from build123d import *

# Parameters (mm, degrees)
BOSS_EXTRUDE1_DEPTH = 7.5
FILLET1_R           = 3.75
FILLET2_R           = 3.75


# Some blends are built 0.0001 mm under size
with BuildPart() as part:
    # Sketch2 → Boss-Extrude1 (new body)
    with BuildSketch(Plane(origin=(0, 0, 0), x_dir=(1, 0, 0), z_dir=(0, 1, 0))):
        Polygon((-54.865, 27.5), (-54.865, -27.5), (-47.365, -27.5), (-47.365, -5), (47.365, -5), (47.365, -27.5), (54.865, -27.5), (54.865, 27.5), (47.365, 27.5), (47.365, 5), (-47.365, 5), (-47.365, 27.5), align=None)
    extrude(amount=BOSS_EXTRUDE1_DEPTH)

    # Fillet1
    fillet1_edges = [part.edges().sort_by_distance(p)[0] for p in [
        (0, 7.5, 5),
        (-54.865, 0, 0),
        (-47.365, 0, -16.25),
        (0, 0, -5),
        (47.365, 0, -16.25),
        (47.365, 7.5, 16.25),
        (54.865, 0, 0),
        (47.365, 0, 16.25),
        (0, 0, 5),
        (-47.365, 0, 16.25),
        (54.865, 7.5, 0),
        (-54.865, 3.75, 27.5),
        (-54.865, 3.75, -27.5),
        (-47.365, 3.75, -27.5),
        (-47.365, 3.75, -5),
        (47.365, 3.75, -5),
        (47.365, 3.75, -27.5),
        (54.865, 3.75, -27.5),
        (54.865, 3.75, 27.5),
        (47.365, 3.75, 27.5),
        (47.365, 3.75, 5),
        (-47.365, 3.75, 5),
        (-47.365, 3.75, 27.5),
        (47.365, 7.5, -16.25),
        (0, 7.5, -5),
        (-47.365, 7.5, -16.25),
        (-54.865, 7.5, 0),
        (-47.365, 7.5, 16.25),
    ]]
    fillet(fillet1_edges, radius=FILLET1_R - 0.0001)  # a hair under: the kernel refuses the full size

    # Fillet2
    # the kernel refuses this fillet: 3.75 mm, written as the material it takes off along each edge
    with BuildSketch(Plane(origin=(-47.365, 3.75, -23.75), x_dir=(0, 0, -1), z_dir=(0, -1, 0))) as fillet2_piece_1:
        with BuildLine():
            CenterArc((0.0001, -3.7499), 3.7499, 0, 90)
            Line((3.75, -3.7499), (3.75, 0))
            Line((3.75, 0), (0.0001, 0))
        make_face()
    revolve(axis=Axis((-47.365, 3.75, -23.75), (1, 0, 0)), revolution_arc=90, mode=Mode.SUBTRACT)
    with BuildSketch(Plane(origin=(-47.365, 3.75, -23.75), x_dir=(0, -1, 0), z_dir=(0, 0, 1))) as fillet2_piece_2:
        with BuildLine():
            CenterArc((0.0001, -3.7499), 3.7499, 0, 90)
            Line((3.75, -3.7499), (3.75, 0))
            Line((3.75, 0), (0.0001, 0))
        make_face()
    revolve(axis=Axis((-47.365, 3.75, -23.75), (1, 0, 0)), revolution_arc=90, mode=Mode.SUBTRACT)
    with BuildSketch(Plane(origin=(-54.865, 3.75, 23.75), x_dir=(0, 0, 1), z_dir=(0, -1, 0))) as fillet2_piece_3:
        with BuildLine():
            CenterArc((0.0001, -3.7499), 3.7499, 0, 90)
            Line((3.75, -3.7499), (3.75, 0))
            Line((3.75, 0), (0.0001, 0))
        make_face()
    revolve(axis=Axis((-54.865, 3.75, 23.75), (-1, 0, 0)), revolution_arc=90, mode=Mode.SUBTRACT)
    with BuildSketch(Plane(origin=(-54.865, 3.75, 23.75), x_dir=(0, -1, 0), z_dir=(0, 0, -1))) as fillet2_piece_4:
        with BuildLine():
            CenterArc((0.0001, -3.7499), 3.7499, 0, 90)
            Line((3.75, -3.7499), (3.75, 0))
            Line((3.75, 0), (0.0001, 0))
        make_face()
    revolve(axis=Axis((-54.865, 3.75, 23.75), (-1, 0, 0)), revolution_arc=90, mode=Mode.SUBTRACT)
    with BuildSketch(Plane(origin=(47.365, 3.75, 23.75), x_dir=(0, -1, 0), z_dir=(0, 0, -1))) as fillet2_piece_5:
        with BuildLine():
            CenterArc((0.0001, -3.7499), 3.7499, 0, 90)
            Line((3.75, -3.7499), (3.75, 0))
            Line((3.75, 0), (0.0001, 0))
        make_face()
    revolve(axis=Axis((47.365, 3.75, 23.75), (-1, 0, 0)), revolution_arc=90, mode=Mode.SUBTRACT)
    with BuildSketch(Plane(origin=(47.365, 3.75, 23.75), x_dir=(0, 0, 1), z_dir=(0, -1, 0))) as fillet2_piece_6:
        with BuildLine():
            CenterArc((0.0001, -3.7499), 3.7499, 0, 90)
            Line((3.75, -3.7499), (3.75, 0))
            Line((3.75, 0), (0.0001, 0))
        make_face()
    revolve(axis=Axis((47.365, 3.75, 23.75), (-1, 0, 0)), revolution_arc=90, mode=Mode.SUBTRACT)
    with BuildSketch(Plane(origin=(54.865, 3.75, -23.75), x_dir=(0, -1, 0), z_dir=(0, 0, 1))) as fillet2_piece_7:
        with BuildLine():
            CenterArc((0.0001, -3.7499), 3.7499, 0, 90)
            Line((3.75, -3.7499), (3.75, 0))
            Line((3.75, 0), (0.0001, 0))
        make_face()
    revolve(axis=Axis((54.865, 3.75, -23.75), (1, 0, 0)), revolution_arc=90, mode=Mode.SUBTRACT)
    with BuildSketch(Plane(origin=(54.865, 3.75, -23.75), x_dir=(0, 0, -1), z_dir=(0, -1, 0))) as fillet2_piece_8:
        with BuildLine():
            CenterArc((0.0001, -3.7499), 3.7499, 0, 90)
            Line((3.75, -3.7499), (3.75, 0))
            Line((3.75, 0), (0.0001, 0))
        make_face()
    revolve(axis=Axis((54.865, 3.75, -23.75), (1, 0, 0)), revolution_arc=90, mode=Mode.SUBTRACT)
    with BuildSketch(Plane(origin=(-54.865, 3.75, -23.75), x_dir=(0, 1, 0), z_dir=(0, 0, 1))) as fillet2_piece_9:
        with BuildLine():
            CenterArc((0.0001, -3.7499), 3.7499, 0, 90)
            Line((3.75, -3.7499), (3.75, 0))
            Line((3.75, 0), (0.0001, 0))
        make_face()
    revolve(axis=Axis((-54.865, 3.75, -23.75), (-1, 0, 0)), revolution_arc=90, mode=Mode.SUBTRACT)
    with BuildSketch(Plane(origin=(-54.865, 3.75, -23.75), x_dir=(0, 0, -1), z_dir=(0, 1, 0))) as fillet2_piece_10:
        with BuildLine():
            CenterArc((0.0001, -3.7499), 3.7499, 0, 90)
            Line((3.75, -3.7499), (3.75, 0))
            Line((3.75, 0), (0.0001, 0))
        make_face()
    revolve(axis=Axis((-54.865, 3.75, -23.75), (-1, 0, 0)), revolution_arc=90, mode=Mode.SUBTRACT)
    with BuildSketch(Plane(origin=(-47.365, 3.75, 23.75), x_dir=(0, 1, 0), z_dir=(0, 0, -1))) as fillet2_piece_11:
        with BuildLine():
            CenterArc((0.0001, -3.7499), 3.7499, 0, 90)
            Line((3.75, -3.7499), (3.75, 0))
            Line((3.75, 0), (0.0001, 0))
        make_face()
    revolve(axis=Axis((-47.365, 3.75, 23.75), (1, 0, 0)), revolution_arc=90, mode=Mode.SUBTRACT)
    with BuildSketch(Plane(origin=(-47.365, 3.75, 23.75), x_dir=(0, 0, 1), z_dir=(0, 1, 0))) as fillet2_piece_12:
        with BuildLine():
            CenterArc((0.0001, -3.7499), 3.7499, 0, 90)
            Line((3.75, -3.7499), (3.75, 0))
            Line((3.75, 0), (0.0001, 0))
        make_face()
    revolve(axis=Axis((-47.365, 3.75, 23.75), (1, 0, 0)), revolution_arc=90, mode=Mode.SUBTRACT)
    with BuildSketch(Plane(origin=(54.865, 3.75, 23.75), x_dir=(0, 0, 1), z_dir=(0, 1, 0))) as fillet2_piece_13:
        with BuildLine():
            CenterArc((0.0001, -3.7499), 3.7499, 0, 90)
            Line((3.75, -3.7499), (3.75, 0))
            Line((3.75, 0), (0.0001, 0))
        make_face()
    revolve(axis=Axis((54.865, 3.75, 23.75), (1, 0, 0)), revolution_arc=90, mode=Mode.SUBTRACT)
    with BuildSketch(Plane(origin=(54.865, 3.75, 23.75), x_dir=(0, 1, 0), z_dir=(0, 0, -1))) as fillet2_piece_14:
        with BuildLine():
            CenterArc((0.0001, -3.7499), 3.7499, 0, 90)
            Line((3.75, -3.7499), (3.75, 0))
            Line((3.75, 0), (0.0001, 0))
        make_face()
    revolve(axis=Axis((54.865, 3.75, 23.75), (1, 0, 0)), revolution_arc=90, mode=Mode.SUBTRACT)
    with BuildSketch(Plane(origin=(47.365, 3.75, -23.75), x_dir=(0, 0, -1), z_dir=(0, 1, 0))) as fillet2_piece_15:
        with BuildLine():
            CenterArc((0.0001, -3.7499), 3.7499, 0, 90)
            Line((3.75, -3.7499), (3.75, 0))
            Line((3.75, 0), (0.0001, 0))
        make_face()
    revolve(axis=Axis((47.365, 3.75, -23.75), (-1, 0, 0)), revolution_arc=90, mode=Mode.SUBTRACT)
    with BuildSketch(Plane(origin=(47.365, 3.75, -23.75), x_dir=(0, 1, 0), z_dir=(0, 0, 1))) as fillet2_piece_16:
        with BuildLine():
            CenterArc((0.0001, -3.7499), 3.7499, 0, 90)
            Line((3.75, -3.7499), (3.75, 0))
            Line((3.75, 0), (0.0001, 0))
        make_face()
    revolve(axis=Axis((47.365, 3.75, -23.75), (-1, 0, 0)), revolution_arc=90, mode=Mode.SUBTRACT)
    with BuildSketch(Plane(origin=(54.865, 7.5, -27.5), x_dir=(0, 0, 1), z_dir=(-1, 0, 0)), Plane(origin=(47.365, 7.5, 27.5), x_dir=(0, 0, -1), z_dir=(1, 0, 0))) as fillet2_piece_17:
        with BuildLine():
            CenterArc((FILLET2_R, -FILLET2_R), FILLET2_R, 90, 90)
            Line((0, -FILLET2_R), (0, 0))
            Line((0, 0), (FILLET2_R, 0))
        make_face()
    extrude(amount=7.5, mode=Mode.SUBTRACT)
    with BuildSketch(Plane(origin=(54.865, 0, -27.5), x_dir=(0, 0, 1), z_dir=(-1, 0, 0)), Plane(origin=(47.365, 0, 27.5), x_dir=(0, 0, -1), z_dir=(1, 0, 0)), Plane(origin=(-54.865, 0, 27.5), x_dir=(0, 0, -1), z_dir=(1, 0, 0)), Plane(origin=(-54.865, 7.5, 27.5), x_dir=(0, -1, 0), z_dir=(1, 0, 0)), Plane(origin=(-47.365, 0, -27.5), x_dir=(0, 0, 1), z_dir=(-1, 0, 0)), Plane(origin=(-47.365, 7.5, -27.5), x_dir=(0, -1, 0), z_dir=(-1, 0, 0))) as fillet2_piece_18:
        with BuildLine():
            CenterArc((FILLET2_R, FILLET2_R), FILLET2_R, 180, 90)
            Line((0, FILLET2_R), (0, 0))
            Line((0, 0), (FILLET2_R, 0))
        make_face()
    extrude(amount=7.5, mode=Mode.SUBTRACT)


solid = part.part
The listing builds one solid part. Answer for the finished solid, in the listing's coordinates (mm). A direction names the side the tool comes from. Give positions to 0.01 mm unless a question says otherwise; leave off trailing zeros. One line per question, with ' | ' between items. Start each with the question number.
1. For faces 1 (the face through (48.43, 1.13, 16.35)), 2 (the face through (53.8, 1.13, -0.33)), 3 (the face through (48.43, 6.37, -16.14)), 4 (the face through (-0.611, 1.128, -3.931)), 5 (the face through (48.43, 6.37, 16.35)), determine the directions among +Z, -Z, +X, -X, +Y, -Y from which every point of the face is accessible in a straight line to the end or side of a thin tool.
2. Straight lines are drawn through the part: line 1 (X direction, y = 4, z = 20.5); line 2 (X direction, y = 3.25, z = 8.5); line 3 (Z direction, x = -34, y = 4). For each, find the intervals that lie inside material, in ascending order.
3. Given P1, Ø4, axis at x = -26, y = 2, coming from the -Z side; P2, Ø2, axis at y = 5, z = 3, coming from the -X side; P3, Ø1, axis at x = -17.5, z = 5, coming from the +Y side, each flat-ended and moving along its own axis, determine where each tip first touches the part or whether it passes through.
Result:
1) face 1: +Z, -Y | face 2: +Z, -Z, +X, -Y | face 3: -Z, +Y | face 4: -Z, -Y | face 5: +Z, +Y
2) line 1: x = -54.86 to -47.37, 47.37 to 54.86 | line 2: x = -54.83 to -47.39, 47.39 to 54.83 | line 3: z = -4.99 to 4.99
3) P1: stops at z = -5 | P2: stops at x = -54.86 | P3: stops at y = 5.62
